Could you check a few things on this model? Use its own coordinates, in mm. A direction names the side the tool comes from. Coordinates: 2 decimals unless noted, no trailing zeros. Order: outer loops, then holes, each group sorted by start corner. A loop starts at its lowest first (then second) coordinate and runs counter-clockwise, first axis right, second up. Notation, with made-up numbers: (66, 41.25) -> (94, 41.25) arc R16 ccw to (94, 54.25) -> close; hole circle Ø5 at (-26, 56). An arc over 180 degrees is marked (long way). Return JSON: item names as keys, results as strings. Group by question number.
from build123d import *

# Parameters (mm, degrees)
BOSS_EXTRUDE1_DEPTH     = 20
FILLET1_R               = 4
SKETCH2_R               = 2.75
CUT_EXTRUDE1_DEPTH      = 1.5
LPATTERN1_COUNT         = 2
LPATTERN1_PITCH         = 30
CUT_EXTRUDE2_DEPTH      = 35.641016151
CUT_EXTRUDE2_DEPTH_BACK = 35.641016151
WRAP1_DEPTH             = 1


# Read off the part's stored shape, not the designer's step: Wrap1
with BuildPart() as part:
    # Sketch1 → Boss-Extrude1 (new body)
    with BuildSketch(Plane(origin=(0, 0, 0), x_dir=(1, 0, 0), z_dir=(0, 1, 0))):
        with BuildLine():
            Line((-15, -5), (10, -5))
            Line((10, -5), (10, -15))
            ThreePointArc((10, -15), (15, -20), (20, -15))
            Line((20, -15), (20, 0))
            ThreePointArc((20, 0), (18.535533906, 3.535533906), (15, 5))
            Line((15, 5), (-15, 5))
            ThreePointArc((-15, 5), (-20, 0), (-15, -5))
        make_face()
    extrude(amount=BOSS_EXTRUDE1_DEPTH)

    # Fillet1
    fillet1_edges = [part.edges().sort_by_distance(p)[0] for p in [
        (15, 20, 20),
        (20, 20, 7.5),
        (18.535533906, 20, -3.535533906),
        (0, 20, -5),
        (-20, 20, 0),
        (-2.5, 20, 5),
        (10, 20, 10),
    ]]
    fillet(fillet1_edges, radius=FILLET1_R)

    # Sketch2 → Cut-Extrude1 (cut)
    with BuildSketch(Plane.XZ):
        with Locations(Location((-15, 0, 0), (0, 0, 270))):
            Circle(SKETCH2_R)
    cut_extrude1 = extrude(amount=-CUT_EXTRUDE1_DEPTH, mode=Mode.SUBTRACT)

    # LPattern1: Cut-Extrude1 ×2
    with Locations(*[(i * LPATTERN1_PITCH, 0, 0) for i in range(1, LPATTERN1_COUNT)]):
        add(cut_extrude1, mode=Mode.SUBTRACT)

    # Sketch3 → Cut-Extrude2 (cut, two sides: drawn at the far end of the back side and taken through both)
    with BuildSketch(Plane.XY.offset(-CUT_EXTRUDE2_DEPTH_BACK)):
        with BuildLine():
            Line((5, 17), (-5, 17))
            ThreePointArc((-5, 17), (-8, 20), (-5, 23))
            Line((-5, 23), (5, 23))
            ThreePointArc((5, 23), (8, 20), (5, 17))
        make_face()
    extrude(amount=CUT_EXTRUDE2_DEPTH + CUT_EXTRUDE2_DEPTH_BACK, mode=Mode.SUBTRACT)

    # Wrap1 outline → Wrap1 (add)
    with BuildSketch(Plane(origin=(0, 17, 0), x_dir=(1, 0, 0), z_dir=(0, 1, 0))):
        with BuildLine():
            add(Edge.make_bspline(
                [(1.279846376, -2.374028678), (1.334628235, -2.372005919), (1.439423638, -2.368136466), (1.586709387, -2.326690884), (1.715405832, -2.260778282), (1.805401117, -2.180421216), (1.866547055, -2.099402851), (1.91146986, -2.023004422), (1.954343809, -1.931092566), (1.995394653, -1.823787438), (2.03540343, -1.701296934), (2.074075054, -1.563508285), (2.108116131, -1.409568974), (2.130405187, -1.301938193), (2.142025864, -1.245823549)],
                knots=[0, 0, 0, 0, 0.10403341, 0.199011557, 0.288612319, 0.377191825, 0.425797175, 0.481425289, 0.545557079, 0.61863331, 0.699984683, 0.790771883, 0.890916323, 1, 1, 1, 1], degree=3))
            Line((1.279846376, -2.374028678), (-1.19130747, -2.374028678))
            add(Edge.make_bspline(
                [(0.670872017, -0.840374831), (0.598877184, -0.892890897), (0.460407765, -0.993896327), (0.259247648, -1.136582046), (0.079136214, -1.2721954), (-0.085697103, -1.393939001), (-0.231791362, -1.50542791), (-0.360742391, -1.605057789), (-0.471476435, -1.693040171), (-0.650584686, -1.841423278), (-0.895932385, -2.060152678), (-1.093407848, -2.269997081), (-1.19130747, -2.374028678)],
                knots=[0, 0, 0, 0, 0.110593572, 0.212707314, 0.306051588, 0.390379305, 0.467018215, 0.534117187, 0.592614819, 0.642525788, 0.822780058, 1, 1, 1, 1], degree=3))
            add(Edge.make_bspline(
                [(2.414461761, 1.068279015), (2.378068935, 0.984722167), (2.306117333, 0.819523423), (2.171764082, 0.586037142), (2.024257932, 0.364395962), (1.882362056, 0.191285153), (1.756342108, 0.053944192), (1.645356158, -0.054277839), (1.52024596, -0.169630314), (1.380454268, -0.29172845), (1.224880603, -0.419904333), (1.052848506, -0.553709461), (0.868059484, -0.696771215), (0.737896342, -0.79156374), (0.670872017, -0.840374831)],
                knots=[0, 0, 0, 0, 0.10413489, 0.205883221, 0.307528832, 0.408265615, 0.461433854, 0.520606469, 0.585444086, 0.656004792, 0.732803839, 0.815893726, 0.905198979, 1, 1, 1, 1], degree=3))
            add(Edge.make_bspline(
                [(2.569910479, 1.893599528), (2.568142746, 1.81978224), (2.56468278, 1.675300383), (2.535113724, 1.46316539), (2.486055205, 1.260681768), (2.438163447, 1.131975763), (2.414461761, 1.068279015)],
                knots=[0, 0, 0, 0, 0.261979501, 0.512769921, 0.758869279, 1, 1, 1, 1], degree=3))
            add(Edge.make_bspline(
                [(0.249397658, 3.882381579), (0.333852401, 3.880295856), (0.499413602, 3.876207099), (0.741908223, 3.851223526), (0.971759136, 3.80593405), (1.18959295, 3.744264137), (1.393306246, 3.661376278), (1.586046869, 3.564171248), (1.76456817, 3.445680325), (1.930217215, 3.311921517), (2.08021151, 3.165619914), (2.21133761, 3.008910571), (2.322587283, 2.843726724), (2.412544984, 2.66919338), (2.484129314, 2.487396013), (2.533041577, 2.296802227), (2.565160525, 2.098215825), (2.568307798, 1.962639068), (2.569910479, 1.893599528)],
                knots=[0, 0, 0, 0, 0.074102612, 0.14526736, 0.21355926, 0.279416432, 0.343556942, 0.406228654, 0.468492489, 0.531146675, 0.592790073, 0.652016559, 0.710119813, 0.767135501, 0.823967905, 0.881147087, 0.939476717, 1, 1, 1, 1], degree=3))
            add(Edge.make_bspline(
                [(-1.595153624, 3.18366363), (-1.537018416, 3.239488538), (-1.421267077, 3.350639908), (-1.227322021, 3.49323037), (-1.01917847, 3.614849236), (-0.794503481, 3.712369576), (-0.555192573, 3.789539817), (-0.300158666, 3.843743016), (-0.03027423, 3.875864088), (0.154757504, 3.880176079), (0.249397658, 3.882381579)],
                knots=[0, 0, 0, 0, 0.119107626, 0.23715177, 0.355050392, 0.47498588, 0.598670295, 0.726365388, 0.860041186, 1, 1, 1, 1], degree=3))
            add(Edge.make_bspline(
                [(-2.148038239, 1.770202092), (-2.146834557, 1.839213319), (-2.1444639, 1.975131192), (-2.115761448, 2.174024084), (-2.0725438, 2.364349945), (-2.013797101, 2.547053872), (-1.93451202, 2.719957511), (-1.839205925, 2.884783326), (-1.727409324, 3.041427104), (-1.639506749, 3.135963346), (-1.595153624, 3.18366363)],
                knots=[0, 0, 0, 0, 0.132803649, 0.26155729, 0.386082589, 0.508400008, 0.630401232, 0.751619273, 0.874674186, 1, 1, 1, 1], degree=3))
            add(Edge.make_bspline(
                [(-1.208935675, 0.497766194), (-1.274132827, 0.50149434), (-1.401855252, 0.508797847), (-1.58379437, 0.575310486), (-1.747403804, 0.682290997), (-1.890553306, 0.830420443), (-2.008834141, 1.01608116), (-2.088271481, 1.239599951), (-2.141324633, 1.493680029), (-2.145722196, 1.674808207), (-2.148038239, 1.770202092)],
                knots=[0, 0, 0, 0, 0.110139331, 0.215764983, 0.323707128, 0.438906263, 0.562183724, 0.693638164, 0.838649921, 1, 1, 1, 1], degree=3))
            add(Edge.make_bspline(
                [(-0.301884393, 1.369561066), (-0.304766572, 1.30886225), (-0.310374385, 1.190761489), (-0.360035913, 1.021550791), (-0.443342029, 0.869740737), (-0.557930256, 0.738678363), (-0.695194398, 0.631756347), (-0.851287883, 0.551805139), (-1.025431534, 0.507328091), (-1.146729825, 0.50100757), (-1.208935675, 0.497766194)],
                knots=[0, 0, 0, 0, 0.129242333, 0.251464839, 0.372304265, 0.495878621, 0.620081591, 0.741344555, 0.867352775, 1, 1, 1, 1], degree=3))
            add(Edge.make_bspline(
                [(-0.962140803, 2.109945681), (-0.909824085, 2.094806974), (-0.81039346, 2.066035077), (-0.675027986, 2.002430367), (-0.560830979, 1.92712373), (-0.46427764, 1.841406615), (-0.391475884, 1.740340724), (-0.339690156, 1.627067557), (-0.306087178, 1.502350913), (-0.303311641, 1.414655948), (-0.301884393, 1.369561066)],
                knots=[0, 0, 0, 0, 0.151156851, 0.287281401, 0.413669873, 0.530293514, 0.644009236, 0.756908248, 0.874996313, 1, 1, 1, 1], degree=3))
            add(Edge.make_bspline(
                [(-1.348358752, 2.265394399), (-1.330621209, 2.251855949), (-1.288474303, 2.219686679), (-1.202511656, 2.184828621), (-1.092623552, 2.143667428), (-1.00837918, 2.121895451), (-0.962140803, 2.109945681)],
                knots=[0, 0, 0, 0, 0.159109439, 0.378066483, 0.65864549, 1, 1, 1, 1], degree=3))
            add(Edge.make_bspline(
                [(-1.430089521, 2.464112348), (-1.429415195, 2.444204185), (-1.428114492, 2.405803442), (-1.411058666, 2.351977791), (-1.385555484, 2.303870537), (-1.360780125, 2.278243013), (-1.348358752, 2.265394399)],
                knots=[0, 0, 0, 0, 0.268945253, 0.518766978, 0.758729042, 1, 1, 1, 1], degree=3))
            add(Edge.make_bspline(
                [(-0.197717726, 3.369561066), (-0.28241452, 3.365853817), (-0.446198046, 3.358684877), (-0.681222607, 3.303774927), (-0.893632691, 3.209273649), (-1.077682983, 3.0804735), (-1.229219898, 2.93431847), (-1.344105461, 2.782798304), (-1.415738038, 2.624883436), (-1.425407352, 2.516563894), (-1.430089521, 2.464112348)],
                knots=[0, 0, 0, 0, 0.151816317, 0.293576777, 0.429964406, 0.566304914, 0.694365033, 0.806085808, 0.906100976, 1, 1, 1, 1], degree=3))
            add(Edge.make_bspline(
                [(0.928884838, 1.959304656), (0.928086086, 2.015438052), (0.926539001, 2.124161628), (0.911151444, 2.281372808), (0.890291843, 2.428618132), (0.855346146, 2.564724047), (0.815441285, 2.692385245), (0.761060485, 2.807885158), (0.701186968, 2.914806673), (0.629381656, 3.009462922), (0.551801509, 3.095312), (0.463668068, 3.167247991), (0.370794497, 3.230338766), (0.271044111, 3.28236916), (0.163381009, 3.320276983), (0.04991907, 3.349915646), (-0.071775658, 3.365230608), (-0.154947449, 3.36809043), (-0.197717726, 3.369561066)],
                knots=[0, 0, 0, 0, 0.082284271, 0.159374645, 0.231497254, 0.300083139, 0.36523236, 0.427274673, 0.486932074, 0.544586116, 0.60112786, 0.656190593, 0.710940404, 0.765594865, 0.820607428, 0.877984079, 0.93725451, 1, 1, 1, 1], degree=3))
            add(Edge.make_bspline(
                [(0.517025864, 0.374368758), (0.549928586, 0.43914421), (0.615149426, 0.567544204), (0.697152899, 0.765273295), (0.770951673, 0.962291119), (0.827867417, 1.161343452), (0.873192914, 1.360332754), (0.905111682, 1.559455639), (0.92522592, 1.759102273), (0.927663621, 1.892484206), (0.928884838, 1.959304656)],
                knots=[0, 0, 0, 0, 0.131745637, 0.261150462, 0.388067803, 0.513189353, 0.636374668, 0.758087597, 0.878808958, 1, 1, 1, 1], degree=3))
            add(Edge.make_bspline(
                [(-0.805089521, -1.369220985), (-0.723674568, -1.275391825), (-0.566728304, -1.09451429), (-0.344338673, -0.83116064), (-0.144847313, -0.585533161), (0.031128622, -0.358191092), (0.186040311, -0.149965293), (0.317060652, 0.040597284), (0.427968481, 0.211694057), (0.488762816, 0.322742687), (0.517025864, 0.374368758)],
                knots=[0, 0, 0, 0, 0.170005554, 0.327725258, 0.471696803, 0.603008639, 0.721148947, 0.826797124, 0.919478664, 1, 1, 1, 1], degree=3))
            add(Edge.make_bspline(
                [(-2.353166444, -3.319541498), (-2.317411217, -3.262535334), (-2.240300808, -3.139594747), (-2.103504918, -2.950449774), (-1.948026633, -2.736340024), (-1.76326396, -2.505230848), (-1.559031147, -2.249795036), (-1.329305353, -1.9745526), (-1.076183846, -1.67797272), (-0.897762158, -1.474766675), (-0.805089521, -1.369220985)],
                knots=[0, 0, 0, 0, 0.080973991, 0.174630064, 0.280853316, 0.39944862, 0.530692677, 0.674513651, 0.830941638, 1, 1, 1, 1], degree=3))
            Line((-2.353166444, -3.319541498), (-2.353166444, -3.809926113))
            Line((-2.353166444, -3.809926113), (2.467346376, -3.809926113))
            Line((2.467346376, -3.809926113), (2.672474581, -1.245823549))
            Line((2.672474581, -1.245823549), (2.142025864, -1.245823549))
        make_face()
    extrude(amount=WRAP1_DEPTH)


solid = part.part
Q1. I want a section at A-A on y = 6.5. Please give me the cut outline in (x, z).
Q2. I'm going to push flat-ended pins straight in: pin 1 Ø5 at (x, y) = (2.5, 7) entering from +Z; pin 2 Ø3.5 at (x, z) = (15, 0) entering from -Y; pin 3 Ø1.1 at (x, y) = (0, 17.5) entering from -Z. Where does each tip first touch, or does it pass through?
Q3. I need wall thicknesses on line 1 along X through (y, z) = (0.4, 0); line 2 along Z through (x, y) = (4, 2.5); line 3 along X through (y, z) = (16, 7). Which ranges of each line are inside material? Lowest first, please. Write a range as from..to.
Q4. We'd pull the mould along X, two halves only. Please class faces 4 (the flat face through (10, 8, 10)), 5 (the cylindrical face through (-12.273, 0.74, 0.358)), 6 (the flat face through (-12, 20, 0)): pulls with the +X half, pulls with the -X half, needs draft (parallel to the pull), parting line crosses it, or undercut.
Q5. I want a section at B-B on z = 7. Please give me the cut outline in (x, y), and give its area (3 significant figures).
Q6. On a 3-axis mill with a long thin cutter (end or side, diameter ignored), from which of +Z, -Z, +X, -X, +Y, -Y can I reach the whole of each face in a straight line? I mean faces 1 (the cylindrical face through (17.727, 0.74, 0.358)), 2 (the cylindrical face through (11.141, 18.797, 9.654)), 3 (the flat face through (0, 17.5, 3.81)). Say none if no direction works.
Response values:
{
 "1": {"outline": "(-15, -5) -> (15, -5) arc R5 ccw to (20, 0) -> (20, 15) arc R5 ccw to (10, 15) -> (10, 5) -> (-15, 5) arc R5 ccw to start"},
 "2": {"pin 1": "stops at z = 5", "pin 2": "stops at y = 1.5", "pin 3": "stops at z = -4.89"},
 "3": {"line 1": "x = -20..-17.75, -12.25..12.25, 17.75..20", "line 2": "z = -5..5", "line 3": "x = 10..20"},
 "4": {"face 4": "pulls with the -X half", "face 5": "undercut", "face 6": "needs draft"},
 "5": {"outline": "(10, 0) -> (20, 0) -> (20, 16) arc R4 ccw to (16, 20) -> (14, 20) arc R4 ccw to (10, 16) -> close", "area": "193 mm²"},
 "6": {"face 1": "-Y", "face 2": "+Z, -X, +Y", "face 3": "+Z, +Y"}
}
